```python
from build123d import *

# Parameters (mm, degrees)
SKETCH1_R           = 3
BOSS_EXTRUDE1_DEPTH = 57.5
SKETCH2_R           = 5
BOSS_EXTRUDE2_DEPTH = 2.5


with BuildPart() as part:
    # Sketch1 → Boss-Extrude1 (new, symmetric)
    with BuildSketch(Plane.XY):
        Circle(SKETCH1_R)
    extrude(amount=BOSS_EXTRUDE1_DEPTH, both=True)

    # Sketch2 → Boss-Extrude2 (add, symmetric)
    with BuildSketch(Plane.XY.offset(57.5)):
        Circle(SKETCH2_R)
    boss_extrude2 = extrude(amount=BOSS_EXTRUDE2_DEPTH, both=True)

    # Mirror1: Boss-Extrude2 across plane
    add(boss_extrude2.mirror(Plane.XY))


solid = part.part
```
Could you check a few things on this model? Use its own coordinates, in mm. A direction names the side the tool comes from. Coordinates: 2 decimals unless noted, no trailing zeros. Write each loop counter-clockwise with the first axis right and the second up, starting at its lowest first coordinate (ties: lowest second). Pieces come first, ordered by that corner, then holes. Notation, with made-up numbers: (71, 71) - (88, 71) arc R25 cw to (88, 99) - close; hole circle Ø7 at (38.5, 39). An arc over 180 degrees is marked (long way). Use a Markdown table: item, result.
Q1. Please list where these lines run through material, in increasing order: L1, parallel to Z at x = 3, y = -1.25; L2, parallel to Y at x = 0.25, z = -29; L3, parallel to Y at x = -1.5, z = 49.
Geometry check:
| item | result |
|---|---|
| L1 | z = -60 to -55, 55 to 60 |
| L2 | y = -2.99 to 2.99 |
| L3 | y = -2.6 to 2.6 |
Q2. Which directions (+Z, -Z, +X, -X, +Y, -Y) give clear straight access to the entire face, cutting with the end or side of a thin tool? Please do faces 4 (the cylindrical face through (-1.08, -4.88, -57.54)), 5 (the flat face through (-0.1, -3.3, 55)).
Geometry check:
| item | result |
|---|---|
| face 4 | +Z, -Z |
| face 5 | none |
Q3. Imagine slicing it at C-C (z = -16). List the corners of the cut face in (x, y) for me.
Geometry check:
| item | result |
|---|---|
| outline | circle Ø6 at (0, 0) |
Q4. I'm going to push flat-ended pins straight in: pin 1 Ø1 at (y, z) = (1, 9.5) entering from +X; pin 2 Ø6 at (x, z) = (-1.5, -30.5) entering from -Y; pin 3 Ø3 at (y, z) = (-3.5, -32) entering from -X. Where does each tip first touch, or does it pass through?
Geometry check:
| item | result |
|---|---|
| pin 1 | stops at x = 2.96 |
| pin 2 | stops at y = -3 |
| pin 3 | stops at x = -2.24 |
Q5. Thinking about a two-plate mould opening in Z: for faces 1 (the flat face through (-0.1, -3.3, -55)), 2 (the flat face through (0, 0, -60)), 3 (the cylindrical face through (-1.08, -4.88, 57.54)), which applies, +Z half, -Z half, draft (parallel to the pull), parting line (faces both ways), or undercut?
Geometry check:
| item | result |
|---|---|
| face 1 | undercut |
| face 2 | -Z half |
| face 3 | draft |
Q6. Imagine slicing it at A-A (x = 0). List the corners of the cut face in (y, z) for me.
Geometry check:
| item | result |
|---|---|
| outline | (-5, -60) - (5, -60) - (5, -55) - (3, -55) - (3, 55) - (5, 55) - (5, 60) - (-5, 60) - (-5, 55) - (-3, 55) - (-3, -55) - (-5, -55) - close |
